Check sheet for the modelled part. Datum: model origin and axes. Units: mm. A direction names the side the tool comes from. Give positions to 0.01 mm unless a question says otherwise; leave off trailing zeros. Write each loop counter-clockwise with the first axis right and the second up, starting at its lowest first coordinate (ties: lowest second). Pieces come first, ordered by that corner, then holes. Notation, with made-up numbers: M -14.5,78.25 L 15.5,78.25 A35 ccw 15.5,112.25 Z; hole C -9.75,-4 d11. An arc over 180 degrees is marked long. Use CSV: the item, a comma, the result in double quotes. Start each with the question number.
1. Access from +Z, -Z, +X, -X, +Y, -Y to the whole of each face (thin tool, end or side, straight path). Record for faces 1 (the face through (12, 61, 11)), 2 (the face through (-0.3, 38.5, 22.5)), 3 (the face through (0, 16, -30)).
2. Cross-section at C-C, the plane y = 46. Enter the section's corners in (x, z), and give its area (3 significant figures).
3. Cross-section at B-B, the plane y = 62. Enter the section's corners in (x, z), and give its area (3 significant figures).
4. Scan lines: line 1 (Z direction, x = -10, y = 75); line 2 (X direction, y = 34, z = 0); line 3 (Y direction, x = 0, z = -14.25). Record each from-to range of solid material in increasing order.
5. Mould release check, pull along Z, two halves, no side actions. Record for faces 4 (the face through (10.82, 32.661, -26.096)), 5 (the face through (-1.432, 72.906, -18.592)), 6 (the face through (0, 77, -28)): +Z half, -Z half, draft (parallel to the pull), parting line (faces both ways), or undercut.
6. Cross-section at D-D, the plane x = 7.5. State how many separate pieces and enclosed holes the cut face has, and give its area (3 significant figures).
7. Depth check by flat-ended pin: P1, Ø2, axis at y = 25, z = -17.5, coming from the -X side; P2, Ø3.5, axis at x = -2, z = 18.5, coming from the -Y side; P3, Ø1.5, axis at y = 61, z = 17, coming from the +X side; P4, Ø10, axis at x = -20, z = 1, coming from the +Y side. Enter the tip coordinate at first touch or a pass-through.
8. Cross-section at A-A, the plane z = 0. Enter the section's corners in (x, y).
from build123d import *

# Parameters (mm, degrees)
HOLE_WIZARD_M561_D           = 54
HOLE_WIZARD_M561_DEPTH       = 30
HOLE_WIZARD_M561_CSINK_D     = 58
HOLE_WIZARD_M561_CSINK_ANGLE = 90
CUT_EXTRUDE_START            = 28
SKETCH_4_W                   = 66
SKETCH_4_H                   = 33
CUT_EXTRUDE_1_DEPTH          = 67.350410704
CUT_EXTRUDE_START_2          = -28
SKETCH_4_2_W                 = 66
SKETCH_4_2_H                 = 33
CUT_EXTRUDE_2_DEPTH          = 67.350410704
SKETCH_5_R                   = 11
CUT_EXTRUDE_3_DEPTH          = 108.396461767
CUT_EXTRUDE_5_DEPTH          = 50
CUT_EXTRUDE_6_DEPTH          = 95.350410791
CUT_EXTRUDE_6_DEPTH_BACK     = 95.350410791
CHAMFER_1_SIZE               = 1.6
CUT_EXTRUDE_8_DEPTH          = 95.350410791


with BuildPart() as part:
    # Sketch 1 → Revolve 1 (revolve)
    with BuildSketch(Plane.XY, mode=Mode.PRIVATE) as revolve_1_sk:
        with BuildLine():
            Line((-33, 0), (-33, 82))
            Line((-33, 82), (0, 82))
            Line((0, 82), (0, 40))
            Line((0, 40), (-22.5, 40))
            Line((-22.5, 40), (-22.5, 37))
            Line((-22.5, 37), (-27.25, 37))
            ThreePointArc((-27.25, 37), (-27.957106781, 36.707106781), (-28.25, 36))
            Line((-28.25, 36), (-28.25, 29.414213562))
            ThreePointArc((-28.25, 29.414213562), (-28.173879533, 29.03153013), (-27.957106781, 28.707106781))
            Line((-27.957106781, 28.707106781), (0, 0.75))
            Line((0, 0.75), (0, 0))
            Line((0, 0), (-33, 0))
        make_face()
    revolve(revolve_1_sk.sketch.rotate(Axis((0, 0, 0), (0, 1, 0)), 270), axis=Axis((0, 0, 0), (0, 1, 0)))

    # Hole Wizard M561
    with Locations(Plane(origin=(0, 0, 0), x_dir=(-1, 0, 0), z_dir=(0, -1, 0))):
        with Locations((0, 0)):
            CounterSinkHole(HOLE_WIZARD_M561_D / 2, HOLE_WIZARD_M561_CSINK_D / 2, depth=HOLE_WIZARD_M561_DEPTH, counter_sink_angle=HOLE_WIZARD_M561_CSINK_ANGLE)

    # Sketch 4 → Cut-Extrude 1 (cut, through all)
    with BuildSketch(Plane.XY.offset(CUT_EXTRUDE_START)):
        with Locations((0, 65.5)):
            Rectangle(SKETCH_4_W, SKETCH_4_H)
    extrude(amount=CUT_EXTRUDE_1_DEPTH, mode=Mode.SUBTRACT)

    # Sketch 4_2 → Cut-Extrude 2 (cut, through all)
    with BuildSketch(Plane.XY.offset(CUT_EXTRUDE_START_2)):
        with Locations((0, 65.5)):
            Rectangle(SKETCH_4_2_W, SKETCH_4_2_H)
    extrude(amount=-CUT_EXTRUDE_2_DEPTH, mode=Mode.SUBTRACT)

    # Sketch 5 → Cut-Extrude 3 (cut, through all)
    with BuildSketch(Plane.XY.offset(28)):
        with Locations((0, 62)):
            Circle(SKETCH_5_R)
    extrude(amount=-CUT_EXTRUDE_3_DEPTH, mode=Mode.SUBTRACT)

    # Sketch 6 → Cut-Extrude 5 (cut)
    with BuildSketch(Plane(origin=(0, 82, 0), x_dir=(1, 0, 0), z_dir=(0, 1, 0))):
        with BuildLine():
            Line((17.68337521, -11), (-17.68337521, -11))
            ThreePointArc((-17.68337521, -11), (-23.837274331, -11.286764074), (-27, -6))
            Line((-27, -6), (-27, 6))
            ThreePointArc((-27, 6), (-23.837274331, 11.286764074), (-17.68337521, 11))
            Line((-17.68337521, 11), (17.68337521, 11))
            ThreePointArc((17.68337521, 11), (23.837274331, 11.286764074), (27, 6))
            Line((27, 6), (27, -6))
            ThreePointArc((27, -6), (23.837274331, -11.286764074), (17.68337521, -11))
        make_face()
    extrude(amount=-CUT_EXTRUDE_5_DEPTH, mode=Mode.SUBTRACT)

    # Sketch 7 → Cut-Extrude 6 (cut, two sides: drawn at the far end of the back side and taken through both)
    with BuildSketch(Plane.XY.offset(-CUT_EXTRUDE_6_DEPTH_BACK)):
        Polygon((-33, 82), (-18, 82), (-33, 67), align=None)
        Polygon((33, 67), (33, 82), (18, 82), align=None)
    extrude(amount=CUT_EXTRUDE_6_DEPTH + CUT_EXTRUDE_6_DEPTH_BACK, mode=Mode.SUBTRACT)

    # Chamfer 1
    chamfer_1_edges = [part.edges().sort_by_distance(p)[0] for p in [
        (-11, 62, -28),
    ]]
    chamfer(chamfer_1_edges, length=CHAMFER_1_SIZE)

    # Sketch 10 → Cut-Extrude 8 (cut, through all)
    with BuildSketch(Plane.XY):
        with BuildLine():
            Line((-5.5, 0), (5.5, 0))
            Line((5.5, 0), (5.5, 10.5))
            ThreePointArc((5.5, 10.5), (0, 16), (-5.5, 10.5))
            Line((-5.5, 10.5), (-5.5, 0))
        make_face()
    extrude(amount=-CUT_EXTRUDE_8_DEPTH, mode=Mode.SUBTRACT)


solid = part.part
Worked answers:
1,face 1,"+Y, -Y"
1,face 2,"-Y"
1,face 3,"-Z, -Y"
2,outline,"C 0,0 d66; hole M -27,-6 A6 ccw -17.68,-11 L 17.68,-11 A6 ccw 27,-6 L 27,6 A6 ccw 17.68,11 L -17.68,11 A6 ccw -27,6 Z"
2,area,"2,230 mm^2"
3,outline,"M -27,-6 L -27,6 A6 cw -17.68,11 L -11,11 L -11,28 L -17.46,28 A33 ccw -17.46,-28 L -12.6,-28 L -11,-26.4 L -11,-11 L -17.68,-11 A6 cw Z; M 11,-26.4 L 12.6,-28 L 17.46,-28 A33 ccw 17.46,28 L 11,28 L 11,11 L 17.68,11 A6 cw 27,6 L 27,-6 A6 cw 17.68,-11 L 11,-11 Z"
3,area,"1,240 mm^2"
4,line 1,"z = -28 to -11, 11 to 28"
4,line 2,"x = -33 to -28.25, 28.25 to 33"
4,line 3,"y = 40 to 51, 73 to 82"
5,face 4,"undercut"
5,face 5,"draft"
5,face 6,"-Z half"
6,separate pieces,"4"
6,enclosed holes,"0"
6,area,"1,450 mm^2"
7,P1,"stops at x = -28.58"
7,P2,"stops at y = 40"
7,P3,"stops at x = 28.72"
7,P4,"passes through"
8,outline,"M -33,0 L -29,0 L -27,2 L -27,27.75 L -27.96,28.71 A1 cw -28.25,29.41 L -28.25,36 A1 cw -27.25,37 L -27,37 L -27,73 L -33,67 Z; M 27,2 L 29,0 L 33,0 L 33,67 L 27,73 L 27,37 L 27.25,37 A1 cw 28.25,36 L 28.25,29.41 A1 cw 27.96,28.71 L 27,27.75 Z"
